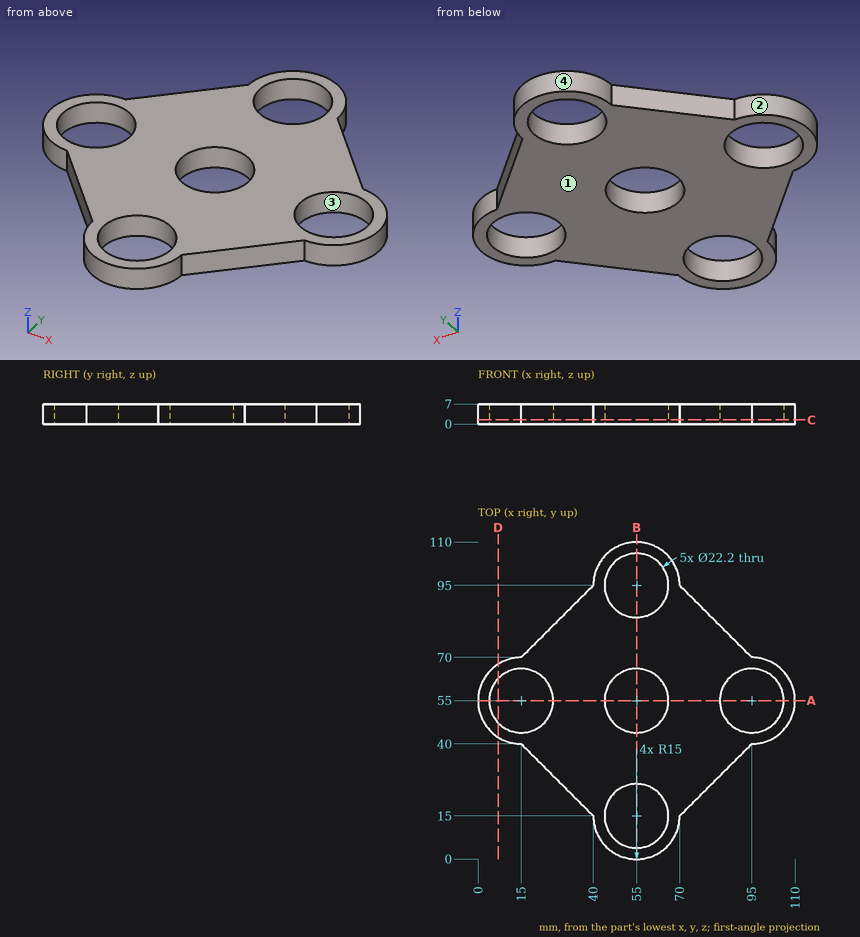
Source: three-view drawing plus pictorial views. Frame: mm from the lowest corner of the part. Give positions to 0.01 mm unless a question says otherwise; leave off trailing zeros. Write each loop counter-clockwise with the first axis right and the second up, starting at its lowest first coordinate (ties: lowest second). Pieces come first, ordered by that corner, then holes. Notation, with made-up numbers: (8.25, 0) -> (48.25, 0) arc R14 ccw to (48.25, 13) -> close; hole circle Ø2 at (89, 27.5). An arc over 180 degrees is marked (long way). Answer in a Markdown table with one row per item.
(1) Draft query along X for the marked faces 1, 2, 3 and 4. Return one class per face: +X half, -X half, draft (parallel to the pull), parting line (faces both ways), or undercut.
Answers below:
| item | result |
|---|---|
| face 1 | draft |
| face 2 | -X half |
| face 3 | undercut |
| face 4 | parting line |
(2) Section query C-C on z = 1.5. Return loops of the section in (x, y), then the cut area to 3 significant figures.
Answers below:
| item | result |
|---|---|
| outline | (15, 40) -> (40, 15) arc R15 ccw to (70, 15) -> (95, 40) arc R15 ccw to (95, 70) -> (70, 95) arc R15 ccw to (40, 95) -> (15, 70) arc R15 ccw to start; hole circle Ø22.2 at (15, 55); hole circle Ø22.2 at (55, 15); hole circle Ø22.2 at (55, 55); hole circle Ø22.2 at (55, 95); hole circle Ø22.2 at (95, 55) |
| area | 4,630 mm^2 |
(3) Section query A-A on y = 55. Return loops of the section in (x, z), then the cut area to 3 significant figures.
Answers below:
| item | result |
|---|---|
| outline | (0, 0) -> (3.9, 0) -> (3.9, 7) -> (0, 7) -> close; (26.1, 0) -> (43.9, 0) -> (43.9, 7) -> (26.1, 7) -> close; (66.1, 0) -> (83.9, 0) -> (83.9, 7) -> (66.1, 7) -> close; (106.1, 0) -> (110, 0) -> (110, 7) -> (106.1, 7) -> close |
| area | 304 mm^2 |
(4) Pin query (flat end, axial travel): pin 1 (18 mm diameter, centred on x = 55, y = 15, fed in from +Z); pin 2 (2 mm diameter, centred on y = 79.5, z = 1.5, fed in from +X); pin 3 (4 mm diameter, centred on x = 47, y = 65.5, fed in from -Z). Return the tip coordinate at first contact, or that it passes through.
Answers below:
| item | result |
|---|---|
| pin 1 | through |
| pin 2 | x = 86.5 |
| pin 3 | z = 0 |
(5) Ray query, line 1 along Y through (x, z) = (55, 3.75); line 2 along X through (y, z) = (95.5, 6); line 3 along Y through (x, z) = (15, 3.75). Return the intervals inside material, ascending. Write a range as [from, to].
Answers below:
| item | result |
|---|---|
| line 1 | [0, 3.9], [26.1, 43.9], [66.1, 83.9], [106.1, 110] |
| line 2 | [40.01, 43.91], [66.09, 69.99] |
| line 3 | [40, 43.9], [66.1, 70] |
(6) Section query D-D on x = 7. Return loops of the section in (y, z).
Answers below:
| item | result |
|---|---|
| outline | (42.31, 0) -> (47.31, 0) -> (47.31, 7) -> (42.31, 7) -> close; (62.69, 0) -> (67.69, 0) -> (67.69, 7) -> (62.69, 7) -> close |
